Part model, mm, in its own coordinate system. Face numbers are marked on the shaded views. Give positions to 0.01 mm unless a question says otherwise; leave off trailing zeros. Write each loop counter-clockwise with the first axis right and the second up, starting at its lowest first coordinate (ties: lowest second). Pieces come first, ordered by that corner, then holes. Notation, with made-up numbers: (13, 89.5) - (59, 89.5) arc R16 cw to (59, 108.5) - close; hole circle Ø11 at (56.25, 42). An arc over 180 degrees is marked (long way). Answer in a Markdown table with one row per item. Add a question column.
1. Band-saw the part on B-B on z = 33. Write the cut outline in (x, y), plus the area to 3 significant figures.
2. Pull direction X, two halves, no side cores. Call the marked faces 1, 2 and 3: released by +X, released by -X, zero draft, split by the parting line, or undercut.
3. Band-saw the part on D-D on x = 177. Write the cut outline in (y, z), plus the area to 3 significant figures.
4. Probe line 1 along Z through (x, y) = (-28, -90.5); line 2 along X through (y, z) = (-76, -336.5); line 3 along X through (y, z) = (-100, -280.5). List the from-to ranges inside material, lowest first.
5. Band-saw the part on A-A on z = -265.5. Write the cut outline in (x, y).
6. Band-saw the part on C-C on y = 128. Write the cut outline in (x, z), plus the area to 3 significant figures.
7. Drop flat-ended pins along their axis: pin 1 Ø4 at (y, z) = (-75, -177.5) entering from +X; pin 2 Ø6 at (x, z) = (342.5, -528.5) entering from -Y; pin 3 Ø11.5 at (y, z) = (379.5, -340) entering from +X. Give the stop position or say it passes through.
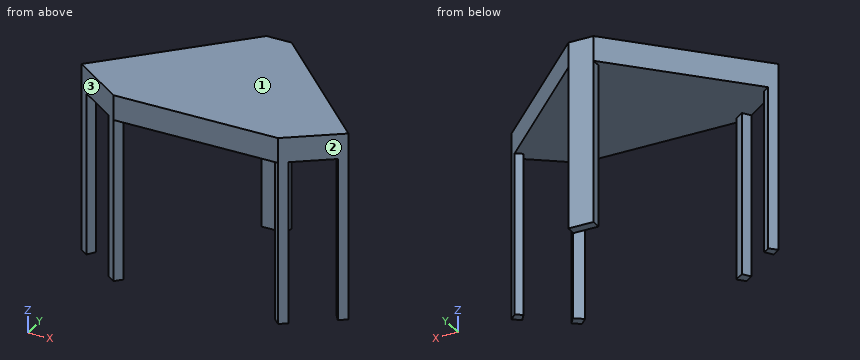
```python
from build123d import *

# Parameters (mm, degrees)
F1_DEPTH = 101.6
F2_W     = 101.6
F2_H     = 38.1
F3_DEPTH = 762
F4_W     = 177.4056817709
F4_H     = 660.4
F5_DEPTH = 76.2


# Not quite as in the source:
# - a pattern or mirror of a feature is missing from the dataset's text; its kind, count and spacing are read off the source's solid


with BuildPart() as f1:
    # F0 (on Top) → F1 (new body)
    with BuildSketch(Plane.XY):
        Polygon((332.1480994978, 125.0519005022), (228.6, 228.6), (0, 228.6), (-228.6, 228.6), (-332.1480994978, 125.0519005022), (-332.1480994978, -228.6), (-228.6, -228.6), (228.6, -228.6), (332.1480994978, -228.6), align=None)
        Polygon((-228.6, 228.6), (0, 228.6), (0, 406.4), (-50.8, 406.4), align=None)
        Polygon((0, 228.6), (228.6, 228.6), (50.8, 406.4), (0, 406.4), align=None)
        Polygon((538.8153672641, -81.6153672641), (332.1480994978, 125.0519005022), (332.1480994978, -228.6), align=None)
        Polygon((-332.1480994978, -228.6), (-332.1480994978, 125.0519005022), (-538.8153672641, -81.6153672641), align=None)
    extrude(amount=F1_DEPTH)

    # F2 (on face) → F3 (join)
    with BuildSketch(Plane.XY.offset(101.6)):
        Polygon((-511.8745989009, -54.6745989009), (-538.8153672641, -81.6153672641), (-332.1480994978, -228.6), (-305.2073311346, -201.6592316368), align=None)
        Polygon((305.2073311346, -201.6592316368), (332.1480994978, -228.6), (538.8153672641, -81.6153672641), (511.8745989009, -54.6745989009), align=None)
        with Locations((0, 387.35)):
            Rectangle(F2_W, F2_H)
    extrude(amount=-F3_DEPTH)

    # F4 (on face) → F5 (cut)
    with BuildSketch(Plane(origin=(219.5423321657, -308.6867865247, 0), x_dir=(0.8149157634, 0.5795794152, 0), z_dir=(0.5795794152, -0.8149157634, 0))):
        with Locations((264.983708636, -330.2)):
            Rectangle(F4_W, F4_H)
    f5 = extrude(amount=-F5_DEPTH, mode=Mode.SUBTRACT)

    # F5_copies: F5 across plane
    add(f5.mirror(Plane(origin=(0, 0, 0), x_dir=(0, 0, -1), z_dir=(-1, 0, 0))), mode=Mode.SUBTRACT)


solid = f1.part
```
Values:
| question | item | result |
|---|---|---|
| 1 | outline | (-538.82, -81.62) - (-332.15, -228.6) - (332.15, -228.6) - (538.82, -81.62) - (50.8, 406.4) - (-50.8, 406.4) - close |
| 1 | area | 416,000 mm² |
| 2 | face 1 | zero draft |
| 2 | face 2 | released by +X |
| 2 | face 3 | released by -X |
| 3 | outline | (-228.6, 0) - (280.2, 0) - (280.2, 101.6) - (-228.6, 101.6) - close |
| 3 | area | 51,700 mm² |
| 4 | line 1 | z = 0 to 101.6 |
| 4 | line 2 | x = -533.2 to -488.07, 488.07 to 533.2 |
| 4 | line 3 | x = -512.97 to -505.14, 505.14 to 512.97 |
| 5 | outline | (-538.82, -81.62) - (-507.77, -103.7) - (-485.99, -73.08) - (-511.87, -54.67) - close; (-363.2, -206.52) - (-332.15, -228.6) - (-305.21, -201.66) - (-341.42, -175.9) - close; (-50.8, 368.3) - (50.8, 368.3) - (50.8, 406.4) - (-50.8, 406.4) - close; (305.21, -201.66) - (332.15, -228.6) - (363.2, -206.52) - (341.42, -175.9) - close; (485.99, -73.08) - (507.77, -103.7) - (538.82, -81.62) - (511.87, -54.67) - close |
| 6 | outline | (-329.2, 0) - (329.2, 0) - (329.2, 101.6) - (-329.2, 101.6) - close |
| 6 | area | 66,900 mm² |
| 7 | pin 1 | stops at x = 534.2 |
| 7 | pin 2 | stops at y = -223.37 |
| 7 | pin 3 | stops at x = 50.8 |
